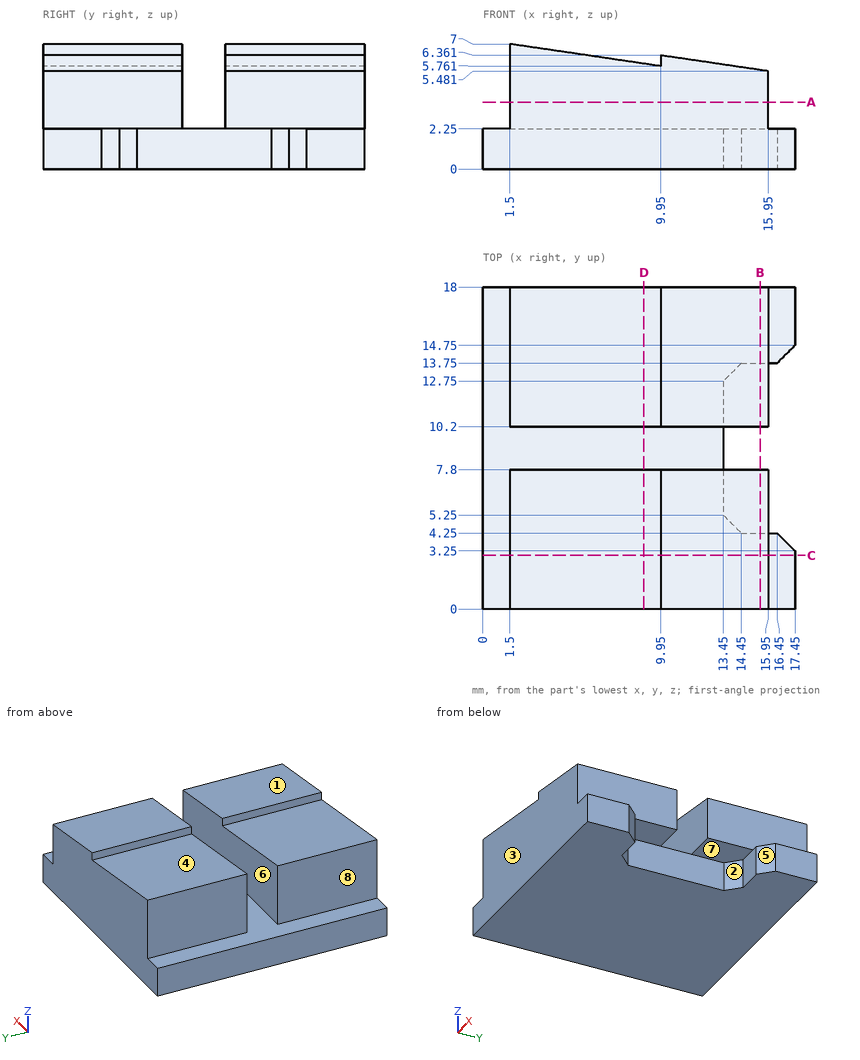
Answer from the drawing. Dimensions are ordinates in mm from the lowest x, y and z of the part. A direction names the side the tool comes from. Give positions to 0.01 mm unless a question says otherwise; leave off trailing zeros. Write each loop counter-clockwise with the first axis right and the second up, starting at its lowest first coordinate (ties: lowest second). Pieces come first, ordered by that corner, then holes. Notation, with made-up numbers: M -38.75,9.5 L -7.75,9.5 A24 ccw -7.75,40.5 Z; hole C -17,20.5 d7. An arc over 180 degrees is marked long. Answer as CSV lines item,"result".
Q1. A cutting plane is placed at D-D on x = 9. Write down the section's boundary in (y, z).
A:
outline,"M 0,0 L 18,0 L 18,5.9 L 10.2,5.9 L 10.2,2.25 L 7.8,2.25 L 7.8,5.9 L 0,5.9 Z"
Q2. The mould has two halves that part along Y. Classify the marked faces 1, 2 and 3: +Y half, -Y half, draft (parallel to the pull), parting line (faces both ways), or undercut.
A:
face 1,"draft"
face 2,"undercut"
face 3,"-Y half"
Q3. A cutting plane is placed at C-C on y = 3. Write down the section's boundary in (x, z), plus the area to 3 significant figures.
A:
outline,"M 0,0 L 17.45,0 L 17.45,2.25 L 15.95,2.25 L 15.95,5.48 L 9.95,6.36 L 9.95,5.76 L 1.5,7 L 1.5,2.25 L 0,2.25 Z"
area,"96.2 mm²"
Q4. A tool of negligible diameter and unlimited length cuts with its end or side. For the marked faces 4, 5, 6, 7 and 8, from which of +Z, -Z, +X, -X, +Y, -Y can it reach the whole face along a straight path? Write none if from no direction.
A:
face 4,"+Z, +Y, -Y"
face 5,"+Z, -Z, +X"
face 6,"+Z, +X, -X"
face 7,"-Z, +X"
face 8,"+Z, -X, +Y, -Y"
Q5. A cutting plane is placed at B-B on x = 15.5. Write down the section's boundary in (y, z).
A:
outline,"M 0,0 L 4.25,0 L 4.25,2.25 L 7.8,2.25 L 7.8,5.55 L 0,5.55 Z; M 10.2,2.25 L 13.75,2.25 L 13.75,0 L 18,0 L 18,5.55 L 10.2,5.55 Z"
Q6. Given P1, Ø2, axis at y = 11.5, z = 5.5, coming from the -X side; P2, Ø1, axis at y = 10, z = 1, coming from the +X side; P3, Ø1.6, axis at y = 13, z = 4, coming from the +X side, each flat-ended and moving along its own axis, determine where each tip first touches the part or whether it passes through.
A:
P1,"stops at x = 1.5"
P2,"stops at x = 13.45"
P3,"stops at x = 15.95"
Q7. Find the intervals of material crossed by probe 1 along Y at (x, z) = (14, 5); probe 2 along X at (y, z) = (14.75, 3.5); probe 3 along Z at (x, y) = (11, 8.5), in increasing order. Write a range as [from, to].
A:
probe 1,"y = [0, 7.8], [10.2, 18]"
probe 2,"x = [1.5, 15.95]"
probe 3,"z = [0, 2.25]"
Q8. A cutting plane is placed at A-A on z = 3.75. Write down the section's boundary in (x, y), plus the area to 3 significant figures.
A:
outline,"M 1.5,0 L 15.95,0 L 15.95,7.8 L 1.5,7.8 Z; M 1.5,10.2 L 15.95,10.2 L 15.95,18 L 1.5,18 Z"
area,"225 mm²"
